from build123d import *

# Parameters (mm, degrees)
BOSS_EXTRUDE1_DEPTH = 58.024
SKETCH2_R           = 3.2
CUT_EXTRUDE1_DEPTH  = 62.780130916
SKETCH4_R           = 1.5
CUT_EXTRUDE2_DEPTH  = 5
CUT_EXTRUDE4_START  = -5
SKETCH5_R           = 1.5
CUT_EXTRUDE4_DEPTH  = 5


with BuildPart() as part:
    # Sketch1 → Boss-Extrude1 (new body)
    with BuildSketch(Plane(origin=(0, 0, 0), x_dir=(0, 0, -1), z_dir=(1, 0, 0))):
        with BuildLine():
            Line((15, -73.484692283), (15, -65.484692283))
            Line((15, -65.484692283), (9.515307717, -60))
            Line((9.515307717, -60), (0, -60))
            Line((0, -60), (-9.515307717, -60))
            Line((-9.515307717, -60), (-15, -65.484692283))
            Line((-15, -65.484692283), (-15, -73.484692283))
            ThreePointArc((-15, -73.484692283), (0, -75), (15, -73.484692283))
        make_face()
    extrude(amount=BOSS_EXTRUDE1_DEPTH)

    # Sketch2 → Cut-Extrude1 (cut, through all)
    with BuildSketch(Plane(origin=(0, -60, 0), x_dir=(1, 0, 0), z_dir=(0, 1, 0))):
        with Locations(Location((29.012, 0, 0), (0, 0, 270))):
            Circle(SKETCH2_R)
    extrude(amount=-CUT_EXTRUDE1_DEPTH, mode=Mode.SUBTRACT)

    # Sketch4 → Cut-Extrude2 (cut)
    with BuildSketch(Plane(origin=(0, 0, 0), x_dir=(0, 0, -1), z_dir=(1, 0, 0))):
        with Locations((0, -66)):
            Circle(SKETCH4_R)
    extrude(amount=CUT_EXTRUDE2_DEPTH, mode=Mode.SUBTRACT)

    # Sketch5 → Cut-Extrude4 (cut)
    with BuildSketch(Plane(origin=(58.024, 0, 0), x_dir=(0, 0, -1), z_dir=(1, 0, 0)).offset(CUT_EXTRUDE4_START)):
        with Locations((0, -66)):
            Circle(SKETCH5_R)
    extrude(amount=CUT_EXTRUDE4_DEPTH, mode=Mode.SUBTRACT)


solid = part.part
Can you work these out from the model? Positions are in its coordinate system, mm. A direction names the side the tool comes from. Coordinates: 2 decimals unless noted, no trailing zeros. Loops run counter-clockwise (first coordinate to the right, second up) from the corner with the lowest first, then second, coordinate; pieces in that order, holes last. Notation, with made-up numbers: (-15.75, 17.5) - (6.25, 17.5) arc R26 cw to (6.25, 48.5) - close; hole circle Ø4 at (35, -13.5). An arc over 180 degrees is marked (long way). Answer as a JSON object with one key per item and string values. Group by question number.
Item 1: For pin 1 (2.5 mm diameter, centred on y = -66, z = 0, fed in from -X); pin 2 (2.5 mm diameter, centred on y = -66, z = 0, fed in from +X); pin 3 (5 mm diameter, centred on y = -63.5, z = 3.5, fed in from -X); pin 4 (8 mm diameter, centred on x = 41, z = 9, fed in from -Y), each with a flat end and sliding along its axis, tell me the tip position at first contact or that it passes through.
Item 2: If we section it at B-B (y = -70): List the corners of the cut face in (x, z) for me.
Item 3: If we section it at A-A (z = 0): List the corners of the cut face in (x, y) for me.
Item 4: If we mould it in two halves opening along Y, with no side actions, what happens to faces 4 (the face through (0, -69, 0)), 5 (the face through (28.606, -74.915, 3.566)), 6 (the face through (5, -66, 0)), 7 (the face through (28.606, -62.704, 12.219))? For each: released by +Y, released by -Y, zero draft, split by the parting line, or undercut.
Item 5: On a 3-axis mill with a long thin cutter (end or side, diameter ignored), from which of +Z, -Z, +X, -X, +Y, -Y can I reach the whole of each face in a straight line? I mean faces 1 (the face through (29, -60, -4)), 2 (the face through (2.465, -64.735, -0.806)), 3 (the face through (53.024, -66, 0)). Say none if no direction works.
Item 6: If I drill on L1, parallel to Y at x = 55, z = 0; L2, parallel to Z at x = 3.15, y = -66; L3, parallel to X at y = -70, z = 0, over which ranges is the centre line in solid material (lowest first)? Write a range as from..to.
Item 7: If we section it at D-D (z = 11): List the corners of the cut face in (x, y) for me, plus the area to 3 significant figures.
Item 8: If we section it at C-C (x = 24): List the corners of the cut face in (y, z) for me, plus the area to 3 significant figures.
Returned:
{
 "1": {"pin 1": "stops at x = 5", "pin 2": "stops at x = 53.02", "pin 3": "stops at x = 0", "pin 4": "stops at y = -74.83"},
 "2": {"outline": "(0, -15) - (58.02, -15) - (58.02, 15) - (0, 15) - close; hole circle Ø6.4 at (29.01, 0)"},
 "3": {"outline": "(0, -75) - (25.81, -75) - (25.81, -60) - (0, -60) - (0, -64.5) - (5, -64.5) - (5, -67.5) - (0, -67.5) - close; (32.21, -75) - (58.02, -75) - (58.02, -67.5) - (53.02, -67.5) - (53.02, -64.5) - (58.02, -64.5) - (58.02, -60) - (32.21, -60) - close"},
 "4": {"face 4": "zero draft", "face 5": "released by -Y", "face 6": "undercut", "face 7": "released by +Y"},
 "5": {"face 1": "+Z, -Z, +X, -X, +Y", "face 2": "-X", "face 3": "+X"},
 "6": {"L1": "y = -75..-67.5, -64.5..-60", "L2": "z = -15..-1.5, 1.5..15", "L3": "x = 0..25.81, 32.21..58.02"},
 "7": {"outline": "(0, -74.19) - (58.02, -74.19) - (58.02, -61.48) - (0, -61.48) - close", "area": "737 mm²"},
 "8": {"outline": "(-73.48, -15) - (-65.48, -15) - (-60, -9.52) - (-60, 9.52) - (-65.48, 15) - (-73.48, 15) arc R75 ccw to start", "area": "405 mm²"}
}
